Study the drawing (mm; zero at the part's minimum x, y, z) and answer. Give positions to 0.01 mm unless a question says otherwise; leave off trailing zeros. Order: outer loops, then holes, each group sorted by start corner. A loop starts at its lowest first (then second) coordinate and runs counter-clockwise, first axis right, second up. Notation, with made-up numbers: (47, 25) - (101, 25) arc R22 cw to (101, 45) - close; hole circle Ø1 at (75, -21). An arc over 180 degrees is marked (long way). Write each question's results on one line, items separated by ' | '. Start each with the question number.
1. Section C-C (z = 46) is taken. Give the vertices of the cut face in (x, y).
2. Determine the mould class of the marked faces 1, 2, 3 and 4 for opening direction Y: released by +Y, released by -Y, zero draft, split by the parting line, or undercut.
3. Section B-B (x = 25.4) is taken. Give the vertices of the cut face in (y, z).
4. Find the intervals of material crossed by L1, parallel to Y at x = 25.4, z = 26; L2, parallel to X at y = 38, z = 17; L3, parallel to Y at x = 30, z = 25, in increasing order.
5. Section A-A (y = 38.1) is taken. Give the vertices of the cut face in (x, z), and give its area (3 significant figures).
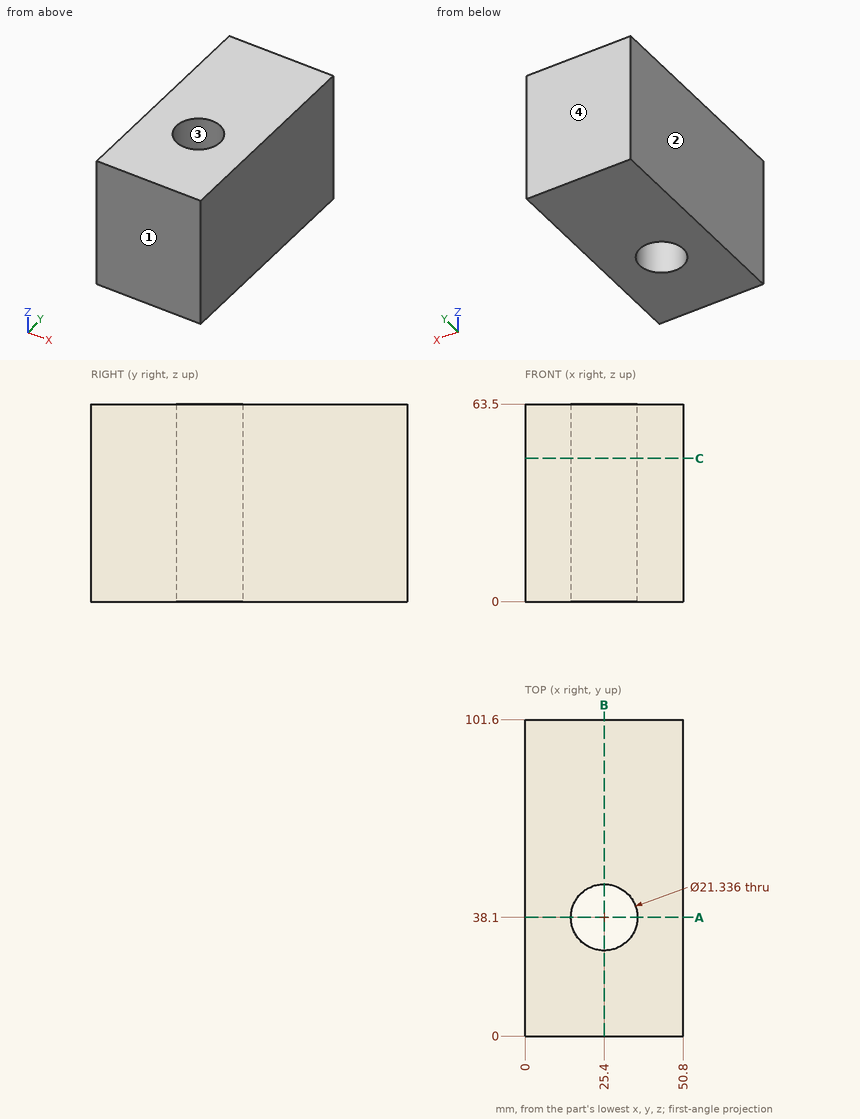
Reported:
1) outline: (0, 0) - (50.8, 0) - (50.8, 101.6) - (0, 101.6) - close; hole circle Ø21.34 at (25.4, 38.1)
2) face 1: released by -Y | face 2: zero draft | face 3: undercut | face 4: released by +Y
3) outline: (0, 0) - (27.43, 0) - (27.43, 63.5) - (0, 63.5) - close; (48.77, 0) - (101.6, 0) - (101.6, 63.5) - (48.77, 63.5) - close
4) L1: 0 to 27.43, 48.77 to 101.6 | L2: 0 to 14.73, 36.07 to 50.8 | L3: 0 to 28.47, 47.73 to 101.6
5) outline: (0, 0) - (14.73, 0) - (14.73, 63.5) - (0, 63.5) - close; (36.07, 0) - (50.8, 0) - (50.8, 63.5) - (36.07, 63.5) - close | area: 1,870 mm²
